Design review of the part built by this model. Coordinates are the model's own, in mm. A direction names the side the tool comes from. Give positions to 0.01 mm unless a question says otherwise; leave off trailing zeros. Write each loop counter-clockwise with the first axis right and the second up, starting at its lowest first coordinate (ties: lowest second). Pieces come first, ordered by that corner, then holes. Notation, with made-up numbers: (-21.5, 51.5) -> (-13.5, 51.5) arc R20 ccw to (-13.5, 58.5) -> close; hole circle Ø6 at (21, 84). An arc over 180 degrees is marked (long way). Put each result on its own line as item: value. Start each with the question number.
from build123d import *

# Parameters (mm, degrees)
ESQUISSE1_R             = 2.2
ESQUISSE1_R_2           = 1.5
ESQUISSE1_R_3           = 2
BOSS_EXTRU_1_DEPTH      = 8
ESQUISSE2_W             = 23.8
ESQUISSE2_H             = 23.3
ENL_V_MAT_EXTRU_1_DEPTH = 2
CONG_1_R                = 2
ENL_V_START             = -2
ESQUISSE4_R             = 3.25
ENL_V_MAT_EXTRU_2_DEPTH = 2
ESQUISSE5_R             = 7.5
ENL_V_MAT_EXTRU_3_DEPTH = 95.836701756
ESQUISSE6_R             = 2
BOSS_EXTRU_2_DEPTH      = 4.5
CONG_2_R                = 6
CONG_3_R                = 6


with BuildPart() as part:
    # Esquisse1 → Boss.-Extru.1 (new body)
    with BuildSketch(Plane(origin=(0, 0, 0), x_dir=(1, 0, 0), z_dir=(0, 1, 0))):
        with BuildLine():
            Line((60, 7), (24, 7))
            ThreePointArc((24, 7), (17.67766953, 17.67766953), (7, 24))
            Line((7, 24), (7, 60))
            ThreePointArc((7, 60), (0, 67), (-7, 60))
            Line((-7, 60), (-7, 24))
            ThreePointArc((-7, 24), (-17.67766953, 17.67766953), (-24, 7))
            Line((-24, 7), (-60, 7))
            ThreePointArc((-60, 7), (-67, 0), (-60, -7))
            Line((-60, -7), (-24, -7))
            ThreePointArc((-24, -7), (-17.67766953, -17.67766953), (-7, -24))
            Line((-7, -24), (-7, -60))
            ThreePointArc((-7, -60), (0, -67), (7, -60))
            Line((7, -60), (7, -24))
            ThreePointArc((7, -24), (17.67766953, -17.67766953), (24, -7))
            Line((24, -7), (60, -7))
            ThreePointArc((60, -7), (67, 0), (60, 7))
        make_face()
        with Locations(Location((14.142135624, 14.142135624, 0), (0, 0, 270))):
            Circle(ESQUISSE1_R, mode=Mode.SUBTRACT)
        with Locations(Location((14.142135624, -14.142135624, 0), (0, 0, 270))):
            Circle(ESQUISSE1_R, mode=Mode.SUBTRACT)
        with Locations(Location((-14.142135624, -14.142135624, 0), (0, 0, 270))):
            Circle(ESQUISSE1_R, mode=Mode.SUBTRACT)
        with Locations(Location((-14.142135624, 14.142135624, 0), (0, 0, 270))):
            Circle(ESQUISSE1_R, mode=Mode.SUBTRACT)
        with Locations(Location((-8, 8, 0), (0, 0, 270))):
            Circle(ESQUISSE1_R_2, mode=Mode.SUBTRACT)
        with Locations(Location((-8, -8, 0), (0, 0, 270))):
            Circle(ESQUISSE1_R_2, mode=Mode.SUBTRACT)
        with Locations(Location((8, -8, 0), (0, 0, 270))):
            Circle(ESQUISSE1_R_2, mode=Mode.SUBTRACT)
        with Locations(Location((8, 8, 0), (0, 0, 270))):
            Circle(ESQUISSE1_R_2, mode=Mode.SUBTRACT)
        with Locations(Location((60, 0, 0), (0, 0, 270))):
            Circle(ESQUISSE1_R_3, mode=Mode.SUBTRACT)
        with Locations(Location((0, -60, 0), (0, 0, 270))):
            Circle(ESQUISSE1_R_3, mode=Mode.SUBTRACT)
        with Locations(Location((-60, 0, 0), (0, 0, 270))):
            Circle(ESQUISSE1_R_3, mode=Mode.SUBTRACT)
        with Locations(Location((0, 60, 0), (0, 0, 270))):
            Circle(ESQUISSE1_R_3, mode=Mode.SUBTRACT)
    extrude(amount=BOSS_EXTRU_1_DEPTH)

    # Esquisse2 → Enlèv. mat.-Extru.1 (cut)
    with BuildSketch(Plane(origin=(0, 8, 0), x_dir=(1, 0, 0), z_dir=(0, 1, 0))):
        Rectangle(ESQUISSE2_W, ESQUISSE2_H)
    extrude(amount=-ENL_V_MAT_EXTRU_1_DEPTH, mode=Mode.SUBTRACT)

    # Congé1
    cong_1_edges = [part.edges().sort_by_distance(p)[0] for p in [
        (-11.9, 7, 11.65),
        (-11.9, 7, -11.65),
        (11.9, 7, -11.65),
        (11.9, 7, 11.65),
    ]]
    fillet(cong_1_edges, radius=CONG_1_R)

    # Esquisse4 → Enlèv. mat.-Extru.2 (cut)
    with BuildSketch(Plane(origin=(0, 6, 0), x_dir=(1, 0, 0), z_dir=(0, 1, 0)).offset(ENL_V_START)):
        with BuildLine():
            Line((-11.9, 9.65), (-11.9, -9.65))
            ThreePointArc((-11.9, -9.65), (-11.314213562, -11.064213562), (-9.9, -11.65))
            Line((-9.9, -11.65), (9.9, -11.65))
            ThreePointArc((9.9, -11.65), (11.314213562, -11.064213562), (11.9, -9.65))
            Line((11.9, -9.65), (11.9, 9.65))
            ThreePointArc((11.9, 9.65), (11.314213562, 11.064213562), (9.9, 11.65))
            Line((9.9, 11.65), (-9.9, 11.65))
            ThreePointArc((-9.9, 11.65), (-11.314213562, 11.064213562), (-11.9, 9.65))
        make_face()
        with Locations(Location((8, 8, 0), (0, 0, 270))):
            Circle(ESQUISSE4_R, mode=Mode.SUBTRACT)
        with Locations(Location((-8, 8, 0), (0, 0, 270))):
            Circle(ESQUISSE4_R, mode=Mode.SUBTRACT)
        with Locations(Location((-8, -8, 0), (0, 0, 270))):
            Circle(ESQUISSE4_R, mode=Mode.SUBTRACT)
        with Locations(Location((8, -8, 0), (0, 0, 270))):
            Circle(ESQUISSE4_R, mode=Mode.SUBTRACT)
    extrude(amount=ENL_V_MAT_EXTRU_2_DEPTH, mode=Mode.SUBTRACT)

    # Esquisse5 → Enlèv. mat.-Extru.3 (cut, through all)
    with BuildSketch(Plane(origin=(0, 4, 0), x_dir=(1, 0, 0), z_dir=(0, 1, 0))):
        with Locations(Location((0, 0, 0), (0, 0, 270))):
            Circle(ESQUISSE5_R)
    extrude(amount=-ENL_V_MAT_EXTRU_3_DEPTH, mode=Mode.SUBTRACT)

    # Esquisse6 → Boss.-Extru.2 (add)
    # profile 1 of 4: a face of its own
    with BuildSketch(Plane(origin=(0, 8, 0), x_dir=(1, 0, 0), z_dir=(0, 1, 0))):
        with BuildLine():
            Line((24, -7), (60, -7))
            ThreePointArc((60, -7), (67, 0), (60, 7))
            Line((60, 7), (24, 7))
            ThreePointArc((24, 7), (25, 0), (24, -7))
        make_face()
        with Locations(Location((60, 0, 0), (0, 0, 270))):
            Circle(ESQUISSE6_R, mode=Mode.SUBTRACT)
    # profile 2 of 4: a face of its own
    with BuildSketch(Plane(origin=(0, 8, 0), x_dir=(1, 0, 0), z_dir=(0, 1, 0))):
        with BuildLine():
            Line((7, 24), (7, 60))
            ThreePointArc((7, 60), (0, 67), (-7, 60))
            Line((-7, 60), (-7, 24))
            ThreePointArc((-7, 24), (0, 25), (7, 24))
        make_face()
        with Locations(Location((0, 60, 0), (0, 0, 270))):
            Circle(ESQUISSE6_R, mode=Mode.SUBTRACT)
    # profile 3 of 4: a face of its own
    with BuildSketch(Plane(origin=(0, 8, 0), x_dir=(1, 0, 0), z_dir=(0, 1, 0))):
        with BuildLine():
            Line((-24, 7), (-60, 7))
            ThreePointArc((-60, 7), (-67, 0), (-60, -7))
            Line((-60, -7), (-24, -7))
            ThreePointArc((-24, -7), (-25, 0), (-24, 7))
        make_face()
        with Locations(Location((-60, 0, 0), (0, 0, 270))):
            Circle(ESQUISSE6_R, mode=Mode.SUBTRACT)
    # profile 4 of 4: a face of its own
    with BuildSketch(Plane(origin=(0, 8, 0), x_dir=(1, 0, 0), z_dir=(0, 1, 0))):
        with BuildLine():
            Line((-7, -24), (-7, -60))
            ThreePointArc((-7, -60), (0, -67), (7, -60))
            Line((7, -60), (7, -24))
            ThreePointArc((7, -24), (0, -25), (-7, -24))
        make_face()
        with Locations(Location((0, -60, 0), (0, 0, 270))):
            Circle(ESQUISSE6_R, mode=Mode.SUBTRACT)
    extrude(amount=BOSS_EXTRU_2_DEPTH)

    # Congé2
    cong_2_edges = [part.edges().sort_by_distance(p)[0] for p in [
        (7, 10.25, 24),
        (-7, 10.25, 24),
        (24, 10.25, -7),
        (24, 10.25, 7),
        (-7, 10.25, -24),
        (7, 10.25, -24),
        (-24, 10.25, 7),
        (-24, 10.25, -7),
    ]]
    fillet(cong_2_edges, radius=CONG_2_R)

    # Congé3
    cong_3_edges = [part.edges().sort_by_distance(p)[0] for p in [
        (7, 4, 24),
        (-7, 4, 24),
        (-24, 4, 7),
        (-24, 4, -7),
        (-7, 4, -24),
        (7, 4, -24),
        (24, 4, -7),
        (24, 4, 7),
    ]]
    fillet(cong_3_edges, radius=CONG_3_R)


solid = part.part
Q1. Mouldability with a two-part tool opening along X and no side actions: class faces 1 (the face through (-46, 12.5, 0)), 2 (the face through (-11.9, 6, 0)), 3 (the face through (67, 6, 0)), 4 (the face through (-7, 6, -44)) as +X half, -X half, draft (parallel to the pull), parting line (faces both ways), or undercut.
Q2. Take a section at C-C on x = 20. Give the boundary of the cut face in (y, z), then the cut area to 3 significant figures.
Q3. Take a section at A-A on y = 10.25. Give the boundary of the cut face in (x, z), then the cut area to 3 significant figures.
Q4. To check wall thickness, follow probe 1 along X at (y, z) = (1.7, 0); probe 2 along X at (y, z) = (8.75, 0); probe 3 along Z at (x, y) = (1, 3.5). State the ranges of each line that lie inside material, in increasing order. Write a range as from..to.
Q5. Take a section at D-D on x = -46. Give the boundary of the cut face in (y, z).
Q6. Take a section at B-B on z = -14. Give the boundary of the cut face in (x, y).
Q7. For pin 1 (7 mm diameter, centred on x = 9, z = -6.5, fed in from +Y); pin 2 (4 mm diameter, centred on x = -48, y = 9.5, fed in from +Z); pin 3 (4.5 mm diameter, centred on y = 5.5, z = -3.5, fed in from -X), all flat-tipped, find the tip position at first contact; note any pin that passes through.
Q8. Machinability: for faces 5 (the face through (0, 6, -11.65)), 6 (the face through (-17.59, 3.944, -17.765)), 7 (the face through (7, 6, 44)), which of the approach directions +Z, -Z, +X, -X, +Y, -Y give a long, thin tool a straight path to every point of the face, cutting with its end or side? Answer none if there is none.
Result:
1. face 1: draft
1. face 2: undercut
1. face 3: +X half
1. face 4: -X half
2. outline: (0, -15) -> (8, -15) -> (8, 15) -> (0, 15) -> close
2. area: 240 mm^2
3. outline: (-60, -7) -> (-30.98, -7) arc R6 ccw to (-24.99, -0.81) arc R25 cw to (-24.99, 0.81) arc R6 ccw to (-30.98, 7) -> (-60, 7) arc R7 ccw to start; (-7, -60) arc R7 ccw to (7, -60) -> (7, -30.98) arc R6 ccw to (0.81, -24.99) arc R25 cw to (-0.81, -24.99) arc R6 ccw to (-7, -30.98) -> close; (-7, 30.98) arc R6 ccw to (-0.81, 24.99) arc R25 cw to (0.81, 24.99) arc R6 ccw to (7, 30.98) -> (7, 60) arc R7 ccw to (-7, 60) -> close; (24.99, -0.81) arc R6 ccw to (30.98, -7) -> (60, -7) arc R7 ccw to (60, 7) -> (30.98, 7) arc R6 ccw to (24.99, 0.81) arc R25 cw to start; hole circle Ø4 at (-60, 0); hole circle Ø4 at (0, -60); hole circle Ø4 at (0, 60); hole circle Ø4 at (60, 0)
3. area: 2,160 mm^2
4. probe 1: x = -67..-62, -58..-7.5, 7.5..58, 62..67
4. probe 2: x = -67..-62, -58..-25, 25..58, 62..67
4. probe 3: z = -66.93..-61.73, -58.27..-7.43, 7.43..58.27, 61.73..66.93
5. outline: (0, -7) -> (12.5, -7) -> (12.5, 7) -> (0, 7) -> close
6. outline: (-20.71, 0) -> (-16.34, 0) -> (-16.34, 8) -> (-20.71, 8) -> close; (-11.95, 0) -> (11.95, 0) -> (11.95, 8) -> (-11.95, 8) -> close; (16.34, 0) -> (20.71, 0) -> (20.71, 8) -> (16.34, 8) -> close
7. pin 1: stops at y = 8
7. pin 2: stops at z = 7
7. pin 3: stops at x = -66.89
8. face 5: +Y
8. face 6: -Z, -X, +Y, -Y
8. face 7: +Z, +X, +Y, -Y
